Geometry check sheet. Reference: the model listing, model coordinates, mm. Coordinates: 2 decimals unless noted, no trailing zeros. Write each loop counter-clockwise with the first axis right and the second up, starting at its lowest first coordinate (ties: lowest second). Pieces come first, ordered by that corner, then holes.
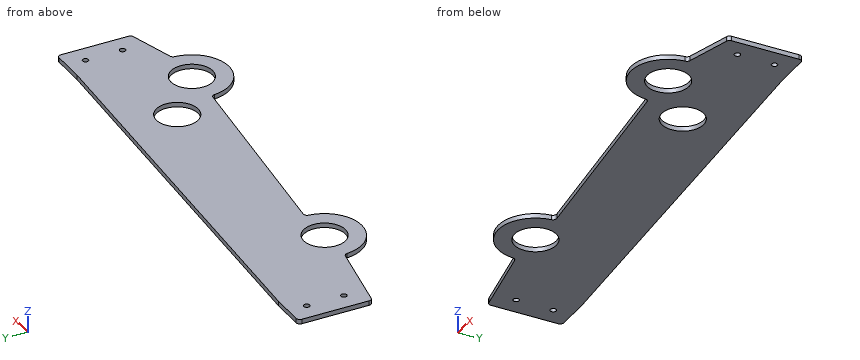
from build123d import *

# Parameters (mm, degrees)
SKETCH1_R           = 14.2875
SKETCH1_R_2         = 2.0193
BOSS_EXTRUDE1_DEPTH = 3.175
FILLET1_R           = 2.54
SKETCH2_R           = 14.2875
CUT_EXTRUDE1_DEPTH  = 238.443914509


with BuildPart() as part:
    # Sketch1 → Boss-Extrude1 (new body)
    with BuildSketch(Plane.XY):
        with BuildLine():
            Line((-146.05, 164.23894), (-171.45, 164.23894))
            Line((-171.45, 164.23894), (-171.45, 113.43894))
            Line((-171.45, 113.43894), (-116.081416722, 103.131947821))
            ThreePointArc((-116.081416722, 103.131947821), (-90.681416722, 77.731947821), (-65.281416722, 103.131947821))
            Line((-65.281416722, 103.131947821), (86.42489431, 86.355953292))
            ThreePointArc((86.42489431, 86.355953292), (111.82489431, 60.955953292), (137.22489431, 86.355953292))
            Line((137.22489431, 86.355953292), (171.45, 96.16694))
            Line((171.45, 96.16694), (171.45, 146.96694))
            Line((171.45, 146.96694), (146.05, 146.96694))
            Line((146.05, 146.96694), (-146.05, 164.23894))
        make_face()
        with Locations((-90.681416722, 103.131947821)):
            Circle(SKETCH1_R, mode=Mode.SUBTRACT)
        with Locations((111.82489431, 86.355953292)):
            Circle(SKETCH1_R, mode=Mode.SUBTRACT)
        with Locations((-158.75, 151.53894)):
            Circle(SKETCH1_R_2, mode=Mode.SUBTRACT)
        with Locations((158.75, 134.26694)):
            Circle(SKETCH1_R_2, mode=Mode.SUBTRACT)
        with Locations((158.75, 108.86694)):
            Circle(SKETCH1_R_2, mode=Mode.SUBTRACT)
        with Locations((-158.75, 126.13894)):
            Circle(SKETCH1_R_2, mode=Mode.SUBTRACT)
    extrude(amount=BOSS_EXTRUDE1_DEPTH)

    # Fillet1
    # the kernel refuses this fillet: 2.54 mm, written as the material it adds along each edge
    with BuildSketch(Plane(origin=(-65.281416722, 103.131947821, 0), x_dir=(-0.05054020357066893, -0.9987220273044123, 0), z_dir=(0, 0, 1))) as fillet1_piece_1:
        with BuildLine():
            CenterArc((2.695814458, 2.536753949), FILLET1_R, 176.586727967, 90.516297483)
            Line((0.160320257, 2.687979466), (0, 0))
            ThreePointArc((0, 0), (1.283721171, 0.032460506), (2.567442341, 0))
        make_face()
    extrude(amount=3.175)
    with BuildSketch(Plane(origin=(-116.081416722, 103.131947821, 0), x_dir=(-0.983111332758604, 0.1830084899713721, 0), z_dir=(0, 0, 1))) as fillet1_piece_2:
        with BuildLine():
            CenterArc((2.028421781, 2.54), FILLET1_R, 194.908754381, 75.091245619)
            ThreePointArc((-0.42607364, 1.886507669), (-0.195074838, 0.947310604), (0, 0))
            Line((0, 0), (2.028421781, 0))
        make_face()
    extrude(amount=3.175)
    with BuildSketch(Plane(origin=(146.05, 146.96694, 0), x_dir=(1, 0, 0), z_dir=(0, 0, 1))) as fillet1_piece_3:
        with BuildLine():
            CenterArc((FILLET1_R * 0.0295394194537, FILLET1_R), FILLET1_R, 266.616015906, 3.383984094)
            Line((-FILLET1_R * 0.0294879135427, FILLET1_R * 0.00174363314861), (0, 0))
            Line((0, 0), (FILLET1_R * 0.0295394194537, 0))
        make_face()
    extrude(amount=3.175)
    with BuildSketch(Plane(origin=(137.22489431, 86.355953292, 0), x_dir=(0.9612833075503766, 0.275561976014486, 0), z_dir=(0, 0, 1))) as fillet1_piece_4:
        with BuildLine():
            CenterArc((1.844513026, -2.54), FILLET1_R, 90, 70.036589556)
            ThreePointArc((-0.542860523, -1.672793255), (-0.256948075, -0.841096436), (0, 0))
            Line((0, 0), (1.844513026, 0))
        make_face()
    extrude(amount=3.175)
    with BuildSketch(Plane(origin=(86.42489431, 86.355953292, 0), x_dir=(-0.9939413150469867, 0.10991206595577574, 0), z_dir=(0, 0, 1))) as fillet1_piece_5:
        with BuildLine():
            CenterArc((2.180444633, 2.54), FILLET1_R, 191.001176441, 78.998823559)
            ThreePointArc((-0.312878461, 2.055293957), (-0.13540237, 1.03084943), (0, 0))
            Line((0, 0), (2.180444633, 0))
        make_face()
    extrude(amount=3.175)
    # the kernel refuses this fillet: 2.54 mm, written as the material it takes off along each edge
    with BuildSketch(Plane(origin=(-171.45, 113.43894, -5.277017888), x_dir=(0, 1, 0), z_dir=(0, 0, 1))) as fillet1_2_piece_1:
        with BuildLine():
            CenterArc((FILLET1_R * 0.831026439026, -FILLET1_R), FILLET1_R, 90, 79.454954882)
            Line((-FILLET1_R * 0.152084893732, -FILLET1_R * 0.816991510029), (0, 0))
            Line((0, 0), (FILLET1_R * 0.831026439026, 0))
        make_face()
    extrude(amount=13.729035776, mode=Mode.SUBTRACT)
    with BuildSketch(Plane(origin=(-171.45, 164.23894, -6.35), x_dir=(1, 0, 0), z_dir=(0, 0, 1)), Plane(origin=(171.45, 146.96694, -6.35), x_dir=(0, -1, 0), z_dir=(0, 0, 1))) as fillet1_2_piece_2:
        with BuildLine():
            CenterArc((FILLET1_R, -FILLET1_R), FILLET1_R, 90, 90)
            Line((0, -FILLET1_R), (0, 0))
            Line((0, 0), (FILLET1_R, 0))
        make_face()
    extrude(amount=15.875, mode=Mode.SUBTRACT)
    with BuildSketch(Plane(origin=(171.45, 96.16694, -4.78545858), x_dir=(-0.9612833075503753, -0.2755619760144905, 0), z_dir=(0, 0, 1))) as fillet1_2_piece_3:
        with BuildLine():
            CenterArc((FILLET1_R * 0.753615524472, -FILLET1_R), FILLET1_R, 90, 74.004492945)
            Line((-FILLET1_R * 0.207667783079, -FILLET1_R * 0.724438023986), (0, 0))
            Line((0, 0), (FILLET1_R * 0.753615524472, 0))
        make_face()
    extrude(amount=12.745917161, mode=Mode.SUBTRACT)

    # Sketch2 → Cut-Extrude1 (cut, through all)
    with BuildSketch(Plane.XY.offset(3.175)):
        with Locations((76.380709606, 115.23549918)):
            Circle(SKETCH2_R)
    extrude(amount=-CUT_EXTRUDE1_DEPTH, mode=Mode.SUBTRACT)


solid = part.part
1. Sectioned sample at B-B, the plane x = -35. Record the boundary of the cut face in (y, z) (1 decimal).
Computed values:
outline: (99.8, 0) - (157.7, 0) - (157.7, 3.2) - (99.8, 3.2) - close
2. Gauge pin test, flat end, axial feed: pin 1 Ø2.5 at (x, y) = (-158.75, 126.14) entering from -Z. Record the tip position at first contact, or that the pin passes through.
Computed values:
pin 1: passes through
3. Thickness scan on line 1 along Y through (x, z) = (-158.75, 1.8); line 2 along Y through (x, z) = (158.75, 1.25); line 3 along Y through (x, z) = (74.5, 1.5). Record the ranges inside material, lowest first.
Computed values:
line 1: y = 111.07 to 124.12, 128.16 to 149.52, 153.56 to 164.24
line 2: y = 92.53 to 106.85, 110.89 to 132.25, 136.29 to 146.97
line 3: y = 87.67 to 101.07, 129.4 to 151.2
4. Sectioned sample at A-A, the plane x = -94. Record the boundary of the cut face in (y, z) (3 decimals).
Computed values:
outline: (77.95, 0) - (89.235, 0) - (89.235, 3.175) - (77.95, 3.175) - close; (117.029, 0) - (161.161, 0) - (161.161, 3.175) - (117.029, 3.175) - close
